```python
from build123d import *

# Parameters (mm, degrees)
CUT_EXTRUDE1_DEPTH                 = 52.594573358
SOCKET_HEAD_CAP_SCREW1_D           = 6.6
SOCKET_HEAD_CAP_SCREW1_CBORE_D     = 11
SOCKET_HEAD_CAP_SCREW1_CBORE_DEPTH = 6.5
TAP1_D                             = 4.917
TAP1_DEPTH                         = 32.999
TAP1_TIP                           = 1.477215832
CHAMFER1_SIZE                      = 0.5


with BuildPart() as part:
    # Sketch1 → Revolve1 (revolve)
    with BuildSketch(Plane.XY, mode=Mode.PRIVATE) as revolve1_sk:
        Polygon((6.5, 17), (6.5, 12.5), (-17, 12.5), (-17, 17), (-22, 17), (-22, 21), (0, 21), (0, 33), (13, 33), (13, 17), align=None)
    revolve(revolve1_sk.sketch.rotate(Axis((-22, 0, 0), (1, 0, 0)), 90), axis=Axis((-22, 0, 0), (1, 0, 0)))

    # Sketch2 → Cut-Extrude1 (cut, through all)
    with BuildSketch(Plane(origin=(0, 0, 0), x_dir=(0, 0, -1), z_dir=(1, 0, 0))):
        with BuildLine():
            Line((24, 22.649503306), (24, -22.649503306))
            ThreePointArc((24, -22.649503306), (33, 0), (24, 22.649503306))
        make_face()
        with BuildLine():
            Line((-24, 22.649503306), (-24, -22.649503306))
            ThreePointArc((-24, -22.649503306), (-33, 0), (-24, 22.649503306))
        make_face()
    extrude(amount=CUT_EXTRUDE1_DEPTH, mode=Mode.SUBTRACT)

    # Socket Head Cap Screw1 (through all)
    with Locations(Plane(origin=(13, 0, 0), x_dir=(0, 0, -1), z_dir=(1, 0, 0))):
        with Locations((-13.25, 22.9496732), (13.25, -22.9496732), (-13.25, -22.9496732), (13.25, 22.9496732)):
            CounterBoreHole(SOCKET_HEAD_CAP_SCREW1_D / 2, SOCKET_HEAD_CAP_SCREW1_CBORE_D / 2, SOCKET_HEAD_CAP_SCREW1_CBORE_DEPTH)

    # Tap1
    with Locations(Plane(origin=(0, 33, 0), x_dir=(1, 0, 0), z_dir=(0, 1, 0))):
        with Locations((6.5, 0)):
            Hole(TAP1_D / 2, depth=TAP1_DEPTH)
            with Locations((0, 0, -(TAP1_DEPTH + TAP1_TIP / 2))):  # 118° drill point
                Cone(0, TAP1_D / 2, TAP1_TIP, mode=Mode.SUBTRACT)

    # Chamfer1
    chamfer1_edges = [part.edges().sort_by_distance(p)[0] for p in [
        (-22, 0, -21),
    ]]
    chamfer(chamfer1_edges, length=CHAMFER1_SIZE)


solid = part.part
```
Geometry check sheet. Reference: the model listing, model coordinates, mm. A direction names the side the tool comes from. Give positions to 0.01 mm unless a question says otherwise; leave off trailing zeros. Order: outer loops, then holes, each group sorted by start corner. A loop starts at its lowest first (then second) coordinate and runs counter-clockwise, first axis right, second up. Notation, with made-up numbers: (8.5, 30) -> (31.5, 30) arc R23 ccw to (31.5, 48) -> close; hole circle Ø8 at (-19.75, 83). An arc over 180 degrees is marked (long way). Write each question's results on one line, items separated by ' | '. Start each with the question number.
(1) Scan lines: line 1 (Z direction, x = 1.5, y = 25); line 2 (Y direction, x = 10.75, z = -13.25); line 3 (Y direction, x = 2.75, z = 13.25). Record each from-to range of solid material in increasing order.
(2) Sectioned sample at C-C (x = -7). Enter the section's corners in (y, z).
(3) Mould release check, pull along Z, two halves, no side actions. Record for faces 4 (the face through (-19.535, -16.855, -2.213)), 5 (the face through (7, -33, 0)), 6 (the face through (13, 7, 16)): pulls with the +Z half, pulls with the -Z half, needs draft (parallel to the pull), parting line crosses it, or undercut.
(4) Access from +Z, -Z, +X, -X, +Y, -Y to the whole of each face (thin tool, end or side, straight path). Record for faces 1 (the face through (6.5, 23, -17)), 2 (the face through (4.155, 22.484, -0.738)), 3 (the face through (9.48, 32.998, -0.376)).
(5) Gauge pin test, flat ends, axial feed: P1, Ø4, axis at x = 8.5, z = 18, coming from the +Y side; P2, Ø1.5, axis at x = -9.5, y = -17.5, coming from the -Z side; P3, Ø5.5, axis at y = 22.95, z = 13.25, coming from the +X side; P4, Ø5.5, axis at y = -24, z = -13, coming from the +X side. Record the tip position at first contact, or that the pin passes through.
(6) Sectioned sample at B-B (y = 0). Enter the section's corners in (x, z).
(7) Sectioned sample at A-A (z = 0). Enter the section's corners in (x, y).
(8) Sectioned sample at D-D (z = 15.5). Give the number of separate pieces and of enclosed holes in the cut face, plus the area to 3 significant figures.
Answer below:
1) line 1: -21.54 to -15.84, -10.66 to 10.66, 15.84 to 21.54 | line 2: -30.22 to -28.45, -17.45 to -10.65, 10.65 to 17.45, 28.45 to 30.22 | line 3: -30.22 to -26.25, -19.65 to 19.65, 26.25 to 30.22
2) outline: circle Ø42 at (0, 0); hole circle Ø25 at (0, 0)
3) face 4: undercut | face 5: parting line crosses it | face 6: needs draft
4) face 1: +X | face 2: +Y | face 3: +X, -X, +Y
5) P1: y = 28.86 | P2: z = -12.67 | P3: through | P4: x = 6.5
6) outline: (-22, -20.5) -> (-21.5, -21) -> (0, -21) -> (0, -24) -> (13, -24) -> (13, -17) -> (6.5, -17) -> (6.5, -12.5) -> (-17, -12.5) -> (-17, -17) -> (-22, -17) -> close; (-22, 17) -> (-17, 17) -> (-17, 12.5) -> (6.5, 12.5) -> (6.5, 17) -> (13, 17) -> (13, 24) -> (0, 24) -> (0, 21) -> (-21.5, 21) -> (-22, 20.5) -> close
7) outline: (-22, -20.5) -> (-21.5, -21) -> (0, -21) -> (0, -33) -> (13, -33) -> (13, -17) -> (6.5, -17) -> (6.5, -12.5) -> (-17, -12.5) -> (-17, -17) -> (-22, -17) -> close; (-22, 17) -> (-17, 17) -> (-17, 12.5) -> (4.04, 12.5) -> (4.04, 33) -> (0, 33) -> (0, 21) -> (-21.5, 21) -> (-22, 20.5) -> close; (8.96, 17) -> (13, 17) -> (13, 33) -> (8.96, 33) -> close
8) separate pieces: 3 | enclosed holes: 0 | area: 1,030 mm2
